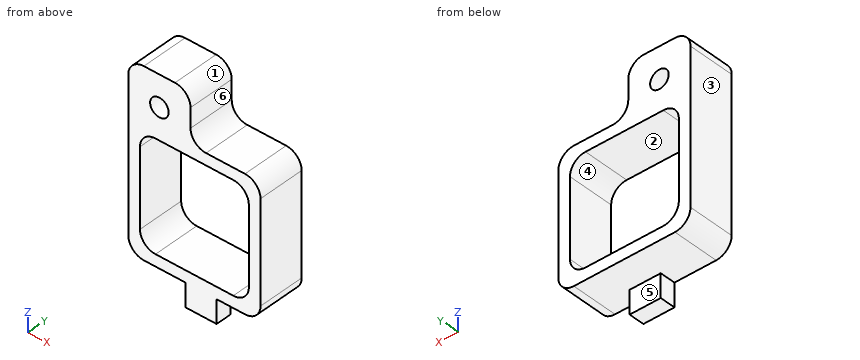
from build123d import *

# Parameters (mm, degrees)
SKETCH1_W             = 8.5
SKETCH1_H             = 8.5
EXTRUDE1_DEPTH        = 3
SKETCH3_W             = 4
SKETCH3_H             = 3
EXTRUDE3_DEPTH        = 3.25
SKETCH2_W             = 7
SKETCH2_H             = 7
EXTRUDE2_DEPTH        = 4
F_0_80_TAPPED_HOLE1_D = 1.19126
SKETCH11_W            = 2
SKETCH11_H            = 1
EXTRUDE5_DEPTH        = 1.5
FILLET1_R             = 1


with BuildPart() as part:
    # Sketch1 → Extrude1 (new body)
    with BuildSketch(Plane(origin=(0, 0, 0), x_dir=(1, 0, 0), z_dir=(0, 1, 0))):
        Rectangle(SKETCH1_W, SKETCH1_H)
    extrude(amount=EXTRUDE1_DEPTH)

    # Sketch3 → Extrude3 (add)
    with BuildSketch(Plane.XY.offset(4.25)):
        with Locations((-2.25, 1.5)):
            Rectangle(SKETCH3_W, SKETCH3_H)
    extrude(amount=EXTRUDE3_DEPTH)

    # Sketch2 → Extrude2 (cut, through all)
    with BuildSketch(Plane(origin=(0, 3, 0), x_dir=(1, 0, 0), z_dir=(0, 1, 0))):
        Rectangle(SKETCH2_W, SKETCH2_H)
    extrude(amount=-EXTRUDE2_DEPTH, mode=Mode.SUBTRACT)

    # #0-80 Tapped Hole1 (through all)
    with Locations(Plane(origin=(-2.25, 3, 5.5), x_dir=(0, 0, 1), z_dir=(0, 1, 0))):
        with Locations((0, 0)):
            Hole(F_0_80_TAPPED_HOLE1_D / 2)

    # Sketch11 → Extrude5 (add)
    with BuildSketch(Plane(origin=(0, 0, -4.25), x_dir=(-1, 0, 0), z_dir=(0, 0, -1))):
        with Locations((-0.42960296, 0.5)):
            Rectangle(SKETCH11_W, SKETCH11_H)
    extrude(amount=EXTRUDE5_DEPTH)

    # Fillet1
    fillet1_edges = [part.edges().sort_by_distance(p)[0] for p in [
        (3.5, 1.5, -3.5),
        (-3.5, 1.5, -3.5),
        (-3.5, 1.5, 3.5),
        (3.5, 1.5, 3.5),
        (-4.25, 1.5, 7.5),
        (-0.25, 1.5, 7.5),
        (-0.25, 1.5, 4.25),
        (4.25, 1.5, 4.25),
        (4.25, 1.5, -4.25),
        (-4.25, 1.5, -4.25),
    ]]
    fillet(fillet1_edges, radius=FILLET1_R)


solid = part.part
Work out the finished part from the listing and answer in its coordinate system (mm). Face numbers are marked on the shaded views. A direction names the side the tool comes from. Give positions to 0.01 mm unless a question says otherwise; leave off trailing zeros. Loops run counter-clockwise (first coordinate to the right, second up) from the corner with the lowest first, then second, coordinate; pieces in that order, holes last. Notation, with made-up numbers: (-20.75, 6) -> (2.25, 6) arc R20 cw to (2.25, 24) -> close; hole circle Ø5 at (18.5, 59). An arc over 180 degrees is marked (long way). Use a Markdown table: item, result. Add a question column.
1. Section D-D on x = -2.25 is taken. Determine the outline of the cut face in (y, z), and give its area (3 significant figures).
2. For the marked faces 4, 5 and 6, determine the directions among +Z, -Z, +X, -X, +Y, -Y from which every point of the face is accessible in a straight line to the end or side of a thin tool.
3. Flat-ended cylindrical pins translate along their axes: pin 1 Ø1 at (x, y) = (3.5, 2.5) entering from +Z; pin 2 Ø3 at (x, z) = (-1, 1.5) entering from +Y; pin 3 Ø1.2 at (x, z) = (0, -5) entering from +Y; pin 4 Ø1.4 at (y, z) = (2, 5.5) entering from +X. Find the tip coordinate at first contact, or state that the pin passes through.
4. Section B-B on x = 2.25 is taken. Determine the outline of the cut face in (y, z), and give its area (3 significant figures).
5. Section C-C on y = 2.05 is taken. Determine the outline of the cut face in (x, z).
6. Determine the mould class of the marked faces 1, 2 and 3 for opening direction Z: released by +Z, released by -Z, zero draft, split by the parting line, or undercut.
7. Find the intervals of material crossed by probe 1 along X at (y, z) = (2.45, 5.5); probe 2 along X at (y, z) = (2.05, 1.75); probe 3 along Z at (x, y) = (-1.5, 2.3), in increasing order.
8. Section A-A on z = -1.5 is taken. Determine the outline of the cut face in (x, y), and give its area (3 significant figures).
Results below:
| question | item | result |
|---|---|---|
| 1 | outline | (0, -4.25) -> (3, -4.25) -> (3, -3.5) -> (0, -3.5) -> close; (0, 3.5) -> (3, 3.5) -> (3, 4.9) -> (0, 4.9) -> close; (0, 6.1) -> (3, 6.1) -> (3, 7.5) -> (0, 7.5) -> close |
| 1 | area | 10.7 mm^2 |
| 2 | face 4 | +Y, -Y |
| 2 | face 5 | -Z, +X, -X, +Y |
| 2 | face 6 | +Z, +X, +Y, -Y |
| 3 | pin 1 | stops at z = 4.25 |
| 3 | pin 2 | passes through |
| 3 | pin 3 | stops at y = 1 |
| 3 | pin 4 | stops at x = -0.14 |
| 4 | outline | (0, -4.25) -> (3, -4.25) -> (3, -3.5) -> (0, -3.5) -> close; (0, 3.5) -> (3, 3.5) -> (3, 4.25) -> (0, 4.25) -> close |
| 4 | area | 4.50 mm^2 |
| 5 | outline | (-4.25, -3.25) arc R1 ccw to (-3.25, -4.25) -> (3.25, -4.25) arc R1 ccw to (4.25, -3.25) -> (4.25, 3.25) arc R1 ccw to (3.25, 4.25) -> (0.75, 4.25) arc R1 cw to (-0.25, 5.25) -> (-0.25, 6.5) arc R1 ccw to (-1.25, 7.5) -> (-3.25, 7.5) arc R1 ccw to (-4.25, 6.5) -> close; hole (-3.5, -2.5) arc R1 ccw to (-2.5, -3.5) -> (2.5, -3.5) arc R1 ccw to (3.5, -2.5) -> (3.5, 2.5) arc R1 ccw to (2.5, 3.5) -> (-2.5, 3.5) arc R1 ccw to (-3.5, 2.5) -> close; hole circle Ø1.19 at (-2.25, 5.5) |
| 6 | face 1 | released by +Z |
| 6 | face 2 | undercut |
| 6 | face 3 | zero draft |
| 7 | probe 1 | x = -4.25 to -2.85, -1.65 to -0.25 |
| 7 | probe 2 | x = -4.25 to -3.5, 3.5 to 4.25 |
| 7 | probe 3 | z = -4.25 to -3.5, 3.5 to 7.5 |
| 8 | outline | (-4.25, 0) -> (-3.5, 0) -> (-3.5, 3) -> (-4.25, 3) -> close; (3.5, 0) -> (4.25, 0) -> (4.25, 3) -> (3.5, 3) -> close |
| 8 | area | 4.50 mm^2 |
